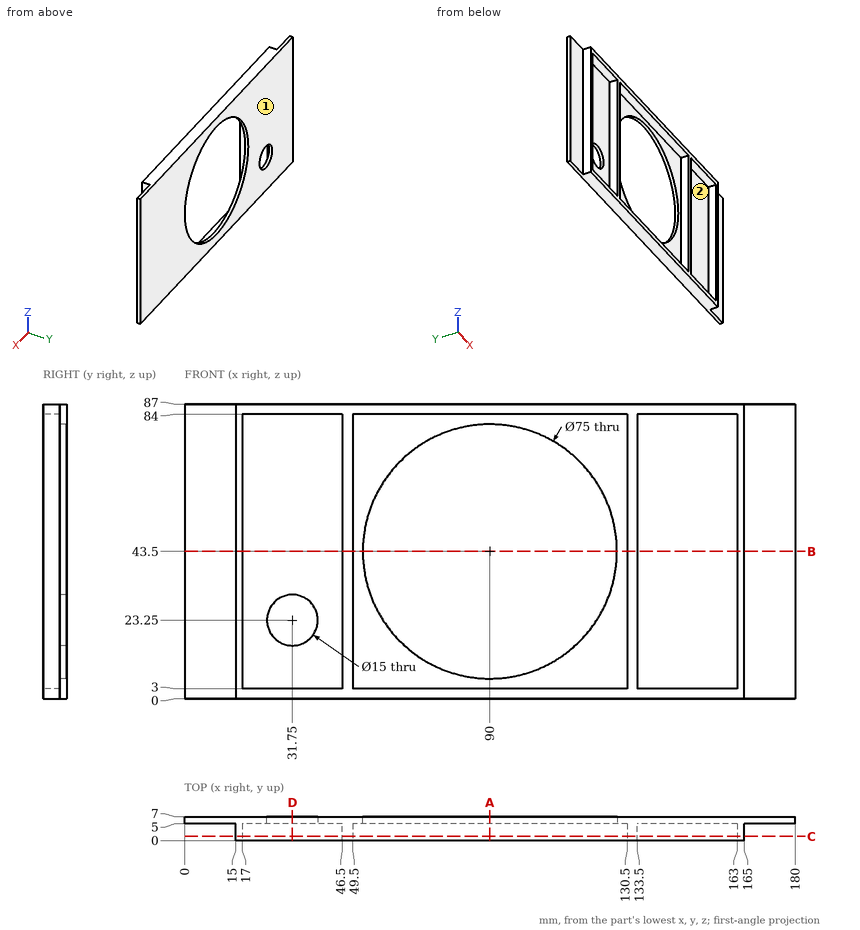
Here's the drawing with two shaded views (mm, measured from the low corner). I have some questions. A direction names the side the tool comes from. Coordinates: 2 decimals unless noted, no trailing zeros. Loops run counter-clockwise (first coordinate to the right, second up) from the corner with the lowest first, then second, coordinate; pieces in that order, holes last. Notation, with made-up numbers: (38, 1.25) -> (62, 1.25) arc R17 ccw to (62, 15.25) -> close; hole circle Ø7 at (10.25, -3). An arc over 180 degrees is marked (long way). Use one line per item in the form item = value. Start each with the question number.
(1) If we section it at A-A (x = 90): Please give me the cut outline in (y, z), then the cut area to 3 significant figures.
(2) Please list where these lines run through material, in increasing order: line 1 along X through (y, z) = (2, 21.5); line 2 along Z through (x, y) = (31.75, 5.5); line 3 along X through (y, z) = (5.75, 43.5).
(3) If we section it at B-B (z = 43.5): Please give me the cut outline in (x, y), then the cut area to 3 significant figures.
(4) If we section it at C-C (y = 1.25): Please give me the cut outline in (x, z), then the cut area to 3 significant figures.
(5) Will these pins go through, and if not, where does the flat tip stop? pin 1 (1.5 mm diameter, centred on y = 3, z = 43, fed in from -X); pin 2 (3 mm diameter, centred on x = 47.5, y = 5.5, fed in from -Z); pin 3 (2.5 mm diameter, centred on y = 1.5, z = 49.5, fed in from +X); pin 4 (1 mm diameter, centred on x = 35.5, z = 71.5, fed in from -Y).
(6) If we section it at D-D (x = 31.75): Please give me the cut outline in (y, z).
(7) On a 3-axis mill with a long thin cutter (end or side, diameter ignored), from which of +Z, -Z, +X, -X, +Y, -Y can I reach the whole of each face in a straight line? I mean the marked faces 1 and 2. Say none if no direction works.
Verdict:
q1.outline = (0, 0) -> (7, 0) -> (7, 6) -> (5, 6) -> (5, 3) -> (0, 3) -> close; (0, 84) -> (5, 84) -> (5, 81) -> (7, 81) -> (7, 87) -> (0, 87) -> close
q1.area = 54.0 mm²
q2.line_1 = 15 to 17, 46.5 to 49.5, 130.5 to 133.5, 163 to 165
q2.line_2 = 0 to 15.75, 30.75 to 87
q2.line_3 = 0 to 52.5, 127.5 to 180
q3.outline = (0, 5) -> (15, 5) -> (15, 0) -> (17, 0) -> (17, 5) -> (46.5, 5) -> (46.5, 0) -> (49.5, 0) -> (49.5, 5) -> (52.5, 5) -> (52.5, 7) -> (0, 7) -> close; (127.5, 5) -> (130.5, 5) -> (130.5, 0) -> (133.5, 0) -> (133.5, 5) -> (163, 5) -> (163, 0) -> (165, 0) -> (165, 5) -> (180, 5) -> (180, 7) -> (127.5, 7) -> close
q3.area = 260 mm²
q4.outline = (15, 0) -> (165, 0) -> (165, 87) -> (15, 87) -> close; hole (17, 3) -> (46.5, 3) -> (46.5, 84) -> (17, 84) -> close; hole (49.5, 3) -> (130.5, 3) -> (130.5, 84) -> (49.5, 84) -> close; hole (133.5, 3) -> (163, 3) -> (163, 84) -> (133.5, 84) -> close
q4.area = 1,710 mm²
q5.pin_1 = 15
q5.pin_2 = 0
q5.pin_3 = 165
q5.pin_4 = 5
q6.outline = (0, 0) -> (7, 0) -> (7, 15.75) -> (5, 15.75) -> (5, 3) -> (0, 3) -> close; (0, 84) -> (5, 84) -> (5, 30.75) -> (7, 30.75) -> (7, 87) -> (0, 87) -> close
q7.face_1 = +Z, -Z, +X, -X, +Y
q7.face_2 = -Y
